Autodesk Inventor part; units mm, degrees
ref_plane "YZ Plane" through (0, 0, 0) normal (1, 0, 0) x (0, 1, 0)
ref_plane "XZ Plane" through (0, 0, 0) normal (0, 1, 0) x (-1, 0, 0)
ref_plane "XY Plane" through (0, 0, 0) normal (0, 0, 1) x (1, 0, 0)
sketch "Sketch1" plane through (0, 0, 0) normal (0, 1, 0) x (-1, 0, 0)
  circle A0 centre (0, 0) radius 101.6
  circle A1 centre (0, 0) radius 76.2
  circle A2 centre (76.2, 0) radius 12.7
  circle A3 centre (38.1, 65.9911) radius 12.7
  circle A4 centre (-38.1, 65.9911) radius 12.7
  circle A5 centre (-76.2, 0) radius 12.7
  circle A6 centre (-38.1, -65.9911) radius 12.7
  circle A7 centre (38.1, -65.9911) radius 12.7
  circle A8 centre (0, 0) radius 38.1
  dimension "d1" = 152.4
  dimension "d0" = 203.2
  dimension "d2" = 25.4
  dimension "d5" = 360
  dimension "d7" = 76.2
extrude "Extrusion1" add sketch "Sketch1" along normal mid plane 25.4 contours A0 | A2 A1 A7 A6 A5 A4 A3
sketch "Sketch2" plane through (0, 12.7, 0) normal (0, 1, 0) x (1, 0, 0)
  circle A0 centre (0, 0) radius 38.1
  circle A1 centre (0, 0) radius 50.8
  dimension "d10" = 101.6
extrude "Extrusion2" add sketch "Sketch2" along normal blind 76.2
properties part number "Leo-Berman-Section-Part-3"
Geometry: final body of the model. Coordinates: model frame, mm. A direction names the side the tool comes from. Coordinates: 2 decimals unless noted, no trailing zeros. Order: outer loops, then holes, each group sorted by start corner. A loop starts at its lowest first (then second) coordinate and runs counter-clockwise, first axis right, second up. Notation, with made-up numbers: M 62,68.25 L 116,68.25 A19 ccw 116,79.25 Z; hole C 79.25,13.25 d11. An arc over 180 degrees is marked long. Answer in a Markdown table with one row per item. Add a question column.
Q1. Line query: L1, parallel to Y at x = 87.5, z = 30.5; L2, parallel to Z at x = -28, y = 4.5; L3, parallel to Z at x = 0, y = 47.5. Output: solid intervals per line, ascending.
Q2. Reachability of faces 1 (the flat face through (-44, -12.7, 1)), 2 (the flat face through (47, 12.7, -21)) from +Z, -Z, +X, -X, +Y, -Y: full face, straight path, thin tool, end or side. Return the list, or none.
Q3. Section query B-B on z = 60. Return the cut outline in (x, y), and give its area (3 significant figures).
Q4. Contact query for flat-ended pins moving along their axis: P1, Ø20.5, axis at x = 38.1, z = 65.99, coming from the -Y side; P2, Ø3, axis at y = 26.5, z = -31.5, coming from the +X side; P3, Ø3, axis at y = 66, z = -48, coming from the -X side; P4, Ø3, axis at x = -66.5, z = -68.5, coming from the +Y side. Output: stop coordinate, or through.
Q5. Section query D-D on x = -43.5. Return the cut outline in (y, z).
Q6. Mould query, pull axis Z, two halves, no side actions, for faces 3 (the cylindrical face through (22.025, 0.178, -99.184)), 4 (the flat face through (7, 88.9, -38)), 5 (the cylindrical face through (64.086, -0.178, -3.815)). Classes: released by +Z, released by -Z, zero draft, split by the parting line, or undercut.
Q7. Section query A-A on x = 0. Return the cut outline in (y, z).
Q8. Section query C-C on z = -24.5. Return the cut outline in (x, y).
Completed:
| question | item | result |
|---|---|---|
| 1 | L1 | y = -12.7 to 12.7 |
| 1 | L2 | z = -97.67 to -73.69, -58.29 to -25.84, 25.84 to 58.29, 73.69 to 97.67 |
| 1 | L3 | z = -50.8 to -38.1, 38.1 to 50.8 |
| 2 | face 1 | +Z, -Z, +X, -X, -Y |
| 2 | face 2 | +Y |
| 3 | outline | M -81.99,-12.7 L -49.3,-12.7 L -49.3,12.7 L -81.99,12.7 Z; M -26.9,-12.7 L 26.9,-12.7 L 26.9,12.7 L -26.9,12.7 Z; M 49.3,-12.7 L 81.99,-12.7 L 81.99,12.7 L 49.3,12.7 Z |
| 3 | area | 3,030 mm2 |
| 4 | P1 | passes through |
| 4 | P2 | stops at x = 41 |
| 4 | P3 | stops at x = -20.45 |
| 4 | P4 | stops at y = 12.7 |
| 5 | outline | M -12.7,-91.82 L 12.7,-91.82 L 12.7,-77.49 L -12.7,-77.49 Z; M -12.7,-54.5 L 12.7,-54.5 L 12.7,-26.24 L 88.9,-26.24 L 88.9,26.24 L 12.7,26.24 L 12.7,54.5 L -12.7,54.5 Z; M -12.7,77.49 L 12.7,77.49 L 12.7,91.82 L -12.7,91.82 Z |
| 6 | face 3 | split by the parting line |
| 6 | face 4 | zero draft |
| 6 | face 5 | undercut |
| 7 | outline | M -12.7,-101.6 L 12.7,-101.6 L 12.7,-50.8 L 88.9,-50.8 L 88.9,-38.1 L -12.7,-38.1 Z; M -12.7,38.1 L 88.9,38.1 L 88.9,50.8 L 12.7,50.8 L 12.7,101.6 L -12.7,101.6 Z |
| 8 | outline | M -98.6,-12.7 L -29.18,-12.7 L -29.18,88.9 L -44.5,88.9 L -44.5,12.7 L -98.6,12.7 Z; M 29.18,-12.7 L 98.6,-12.7 L 98.6,12.7 L 44.5,12.7 L 44.5,88.9 L 29.18,88.9 Z |
